Drawing for the job (mm, zero at the part's lowest x, y, z). A direction names the side the tool comes from. Round coordinates to 2 decimals unless told otherwise and drop trailing zeros. Write each loop counter-clockwise with the first axis right and the second up, starting at its lowest first coordinate (ties: lowest second). Pieces come first, ordered by that corner, then holes. Notation, with made-up numbers: M -21,-10.5 L 19,-10.5 A31 cw 19,20.5 Z; hole C -34.5,-17.75 d10. An arc over 180 degrees is marked long. Use a Markdown table: item, result.
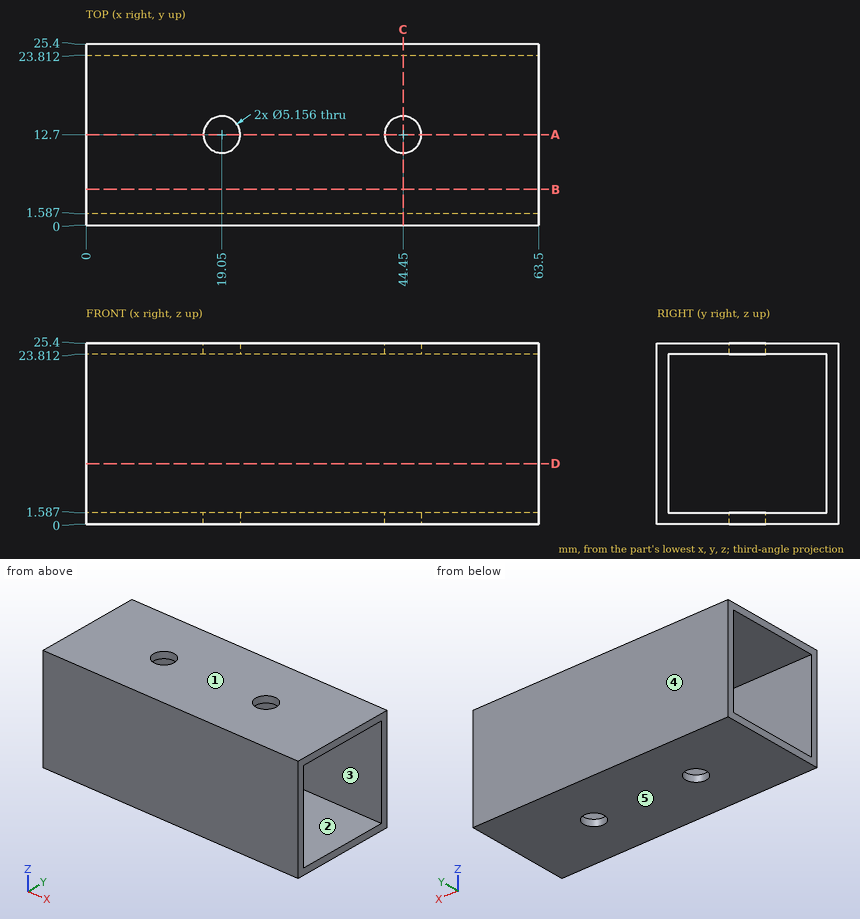
Q1. Cut at B-B on y = 5. Give the cut face in (x, z).
Response values:
| item | result |
|---|---|
| outline | M 0,0 L 63.5,0 L 63.5,1.59 L 0,1.59 Z; M 0,23.81 L 63.5,23.81 L 63.5,25.4 L 0,25.4 Z |
Q2. Two-plate mould, pull along Y, no slides. Class the marked faces 3, 4 and 5: +Y half, -Y half, draft (parallel to the pull), parting line (faces both ways), or undercut.
Response values:
| item | result |
|---|---|
| face 3 | undercut |
| face 4 | +Y half |
| face 5 | draft |
Q3. Drill centre lines: L1, parallel to Z at x = 59, y = 16.25; L2, parallel to Y at x = 44.45, z = 1.05. Where is each one in solid material? Low to high.
Response values:
| item | result |
|---|---|
| L1 | z = 0 to 1.59, 23.81 to 25.4 |
| L2 | y = 0 to 10.12, 15.28 to 25.4 |
Q4. Cut at A-A on y = 12.7. Give the cut face in (x, z), and give its area (3 significant figures).
Response values:
| item | result |
|---|---|
| outline | M 0,0 L 16.47,0 L 16.47,1.59 L 0,1.59 Z; M 0,23.81 L 16.47,23.81 L 16.47,25.4 L 0,25.4 Z; M 21.63,0 L 41.87,0 L 41.87,1.59 L 21.63,1.59 Z; M 21.63,23.81 L 41.87,23.81 L 41.87,25.4 L 21.63,25.4 Z; M 47.03,0 L 63.5,0 L 63.5,1.59 L 47.03,1.59 Z; M 47.03,23.81 L 63.5,23.81 L 63.5,25.4 L 47.03,25.4 Z |
| area | 169 mm2 |
Q5. Which spindle directions (+Z, -Z, +X, -X, +Y, -Y) get a long thin tool onto all of the face, cutting with end or side? Do the marked faces 1 and 2. Say none if no direction does.
Response values:
| item | result |
|---|---|
| face 1 | +Z, +X, -X, +Y, -Y |
| face 2 | +X, -X |
Q6. Cut at C-C on x = 44.45. Give the cut face in (y, z).
Response values:
| item | result |
|---|---|
| outline | M 0,0 L 10.12,0 L 10.12,1.59 L 1.59,1.59 L 1.59,23.81 L 10.12,23.81 L 10.12,25.4 L 0,25.4 Z; M 15.28,0 L 25.4,0 L 25.4,25.4 L 15.28,25.4 L 15.28,23.81 L 23.81,23.81 L 23.81,1.59 L 15.28,1.59 Z |
